For this review, take the finished solid that the model builds, in its own axes (mm). Face numbers are marked on the shaded views. A direction names the side the tool comes from. Give positions to 0.01 mm unless a question says otherwise; leave off trailing zeros. Order: outer loops, then holes, each group sorted by start corner. A loop starts at its lowest first (then second) coordinate and runs counter-clockwise, first axis right, second up. Notation, with made-up numbers: (34, 2.5) - (40, 2.5) arc R34 cw to (40, 32.5) - close; hole circle Ø6 at (-32, 69.25). An arc over 180 degrees is marked (long way). One line per item, written item: value.
```python
from build123d import *

# Parameters (mm, degrees)
SM_BASE_FLANGE_1_DEPTH           = 2
SM_EDGE_FLANGE_1_STRIP_W         = 9.5332
SM_EDGE_FLANGE_1_STRIP_H         = 2
SM_EDGE_FLANGE_1_STRIP_CUT_DEPTH = 20
SM_EDGE_FLANGE_1_DEPTH           = 20
CUT_EXTRUDE_1_DEPTH              = 57.15881498


# Sheet-metal steps are written as plain solids
with BuildPart() as part:
    # Sketch 2 → 基体-法兰1 (new body)
    with BuildSketch(Plane(origin=(0, 0, 0), x_dir=(1, 0, 0), z_dir=(0, 1, 0))):
        with BuildLine():
            Line((-30.031587919, -10), (-25.7014609, -7.5))
            ThreePointArc((-25.7014609, -7.5), (-7.25, 0), (-25.7014609, 7.5))
            Line((-25.7014609, 7.5), (-30.031587919, 10))
            Line((-30.031587919, 10), (-53, 10))
            Line((-53, 10), (-53, -10))
            Line((-53, -10), (-30.031587919, -10))
        make_face()
    extrude(amount=-SM_BASE_FLANGE_1_DEPTH)

    # 边线-法兰1 strip (across the edge) → 边线-法兰1 strip cut (cut)
    with BuildSketch(Plane(origin=(-53, 0, -10), x_dir=(1, 0, 0), z_dir=(0, 0, 1))):
        with Locations((-2, -1)):
            Rectangle(SM_EDGE_FLANGE_1_STRIP_W, SM_EDGE_FLANGE_1_STRIP_H)
    extrude(amount=SM_EDGE_FLANGE_1_STRIP_CUT_DEPTH, mode=Mode.SUBTRACT)

    # 边线-法兰1 section (across the edge) → 边线-法兰1 (add)
    with BuildSketch(Plane(origin=(-53, 0, -10), x_dir=(1, 0, 0), z_dir=(0, 0, 1))):
        with BuildLine():
            Line((0, 0.7666), (0, 11.5))
            Line((0, 11.5), (2, 11.5))
            Line((2, 11.5), (2, 0.7666))
            ThreePointArc((2, 0.7666), (2.224531942, 0.224531942), (2.7666, 0))
            Line((2.7666, 0), (2.7666, -2))
            ThreePointArc((2.7666, -2), (0.810318379, -1.189681621), (0, 0.7666))
        make_face()
    extrude(amount=SM_EDGE_FLANGE_1_DEPTH)

    # 草图10 → 切除-拉伸1 (cut, through all)
    with BuildSketch(Plane(origin=(0, -2, -2), x_dir=(1, 0, 0), z_dir=(0, 1, 0))):
        Polygon((-18, 5.071067812), (-25.071067812, -2), (-18, -9.071067812), (-10.928932188, -2), align=None)
    extrude(amount=CUT_EXTRUDE_1_DEPTH, mode=Mode.SUBTRACT)


solid = part.part
```
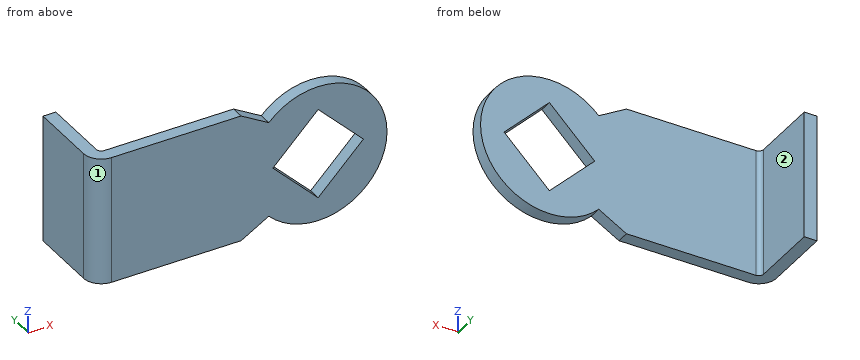
(1) Wall thickness on line 1 (X direction, y = 3, z = 6); line 2 (Y direction, x = -44, z = 0.5); line 3 (Z direction, x = -13, y = -1): over which ranges is each line inside the solid? List them lowest first. Write a range as from..to.
Answers below:
line 1: x = -53..-51
line 2: y = -2..0
line 3: z = -9.52..-2.07, 2.07..9.52
(2) Take a section at D-D (x = -49). Write out the cut boundary in (y, z).
Answers below:
outline: (-2, -10) - (0, -10) - (0, 10) - (-2, 10) - close
(3) For P1, Ø4, axis at x = -33.5, z = -4.5, coming from the +Y side; P2, Ø5, axis at x = -16, y = -0.5, coming from the +Z side; P3, Ø6, axis at x = -14, y = 1.5, coming from the -Z side; P4, Ø4, axis at x = -28, y = 0.5, coming from the -Z side, all flat-tipped, find the tip position at first contact; note any pin that passes through.
Answers below:
P1: stops at y = 0
P2: stops at z = 10.75
P3: stops at z = -10.66
P4: stops at z = -9.95
(4) Take a section at A-A (z = -3). Write out the cut boundary in (x, y), then the cut area to 3 significant figures.
Answers below:
outline: (-53, 0.77) arc R2.77 ccw to (-50.23, -2) - (-22.07, -2) - (-22.07, 0) - (-50.23, 0) arc R0.77 cw to (-51, 0.77) - (-51, 11.5) - (-53, 11.5) - close; (-13.93, -2) - (-7.68, -2) - (-7.68, 0) - (-13.93, 0) - close
area: 95.8 mm^2
(5) Take a section at B-B (x = -21). Write out the cut boundary in (y, z), then the cut area to 3 significant figures.
Answers below:
outline: (-2, -10.32) - (0, -10.32) - (0, -4.07) - (-2, -4.07) - close; (-2, 4.07) - (0, 4.07) - (0, 10.32) - (-2, 10.32) - close
area: 25.0 mm^2
(6) Take a section at C-C (z = 9). Write out the cut boundary in (x, y), then the cut area to 3 significant figures.
Answers below:
outline: (-53, 0.77) arc R2.77 ccw to (-50.23, -2) - (-28.3, -2) - (-28.3, 0) - (-50.23, 0) arc R0.77 cw to (-51, 0.77) - (-51, 11.5) - (-53, 11.5) - close; (-23.88, -2) - (-12.12, -2) - (-12.12, 0) - (-23.88, 0) - close
area: 94.4 mm^2
(7) Machinability: for the marked faces 1 and 2, which of the approach directions +Z, -Z, +X, -X, +Y, -Y give a long, thin tool a straight path to every point of the face, cutting with its end or side? Answer none if there is none.
Answers below:
face 1: +Z, -Z, -X, -Y
face 2: +Z, -Z, +X, +Y
